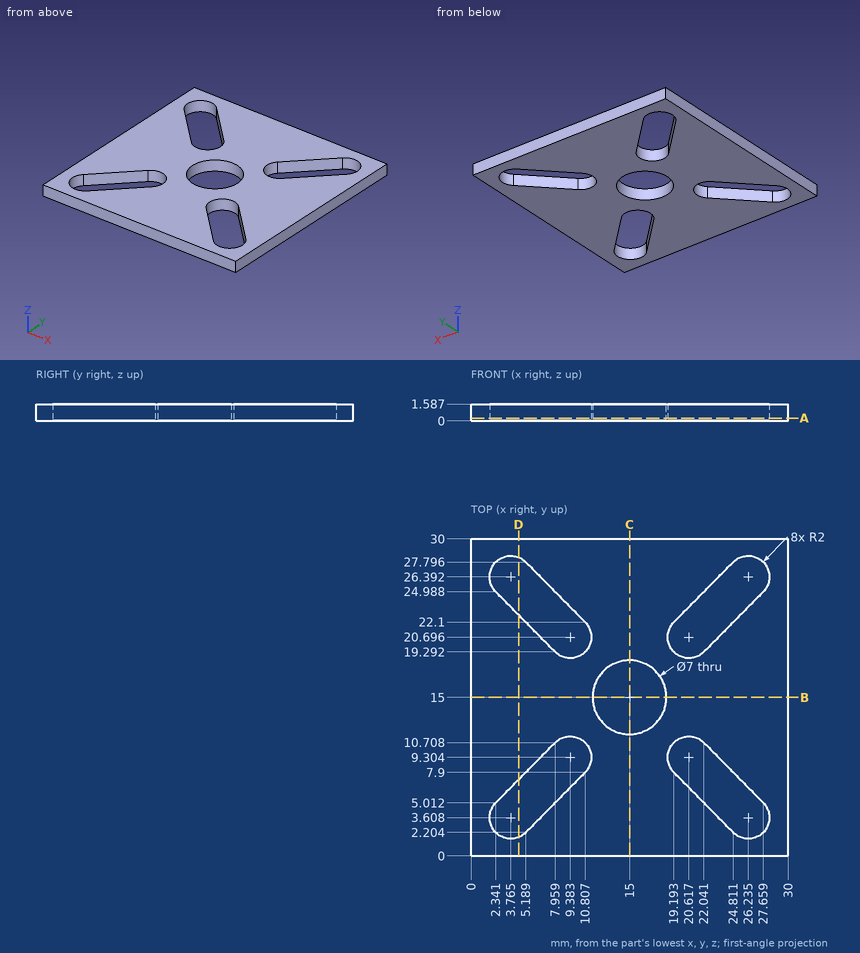
Geometry check sheet. Reference: drawing and pictorial views, mm from the part's lowest x, y, z. Give positions to 0.01 mm unless a question says otherwise; leave off trailing zeros. Write each loop counter-clockwise with the first axis right and the second up, starting at its lowest first coordinate (ties: lowest second). Pieces come first, ordered by that corner, then holes. Notation, with made-up numbers: (45.5, 35) - (58.5, 35) arc R21 ccw to (58.5, 65) - close; hole circle Ø10 at (-32.75, 47). An arc over 180 degrees is marked (long way). Put each result on its own line as item: value.
Q1. Section check B-B on y = 15. Record the cut outline in (x, z).
Result:
outline: (0, 0) - (11.5, 0) - (11.5, 1.59) - (0, 1.59) - close; (18.5, 0) - (30, 0) - (30, 1.59) - (18.5, 1.59) - close
Q2. Scan lines: probe 1 along Y at (x, z) = (15, 0.7); probe 2 along Y at (x, z) = (3.75, 1.45) (1 decimal); probe 3 along X at (y, z) = (9.5, 1.2) (1 decimal). Record each from-to range of solid material in increasing order. Write a range as from..to.
Result:
probe 1: 0..11.5, 18.5..30
probe 2: 0..1.6, 6.4..23.6, 28.4..30
probe 3: 0..6.8, 11.4..18.6, 23.2..30
Q3. Section check D-D on x = 4.5. Record the cut outline in (y, z).
Result:
outline: (0, 0) - (1.75, 0) - (1.75, 1.59) - (0, 1.59) - close; (7.2, 0) - (22.8, 0) - (22.8, 1.59) - (7.2, 1.59) - close; (28.25, 0) - (30, 0) - (30, 1.59) - (28.25, 1.59) - close
Q4. Section check A-A on z = 0.25. Record the cut outline in (x, y) (1 decimal).
Result:
outline: (0, 0) - (30, 0) - (30, 30) - (0, 30) - close; hole (2.3, 5) arc R2 ccw to (5.2, 2.2) - (10.8, 7.9) arc R2 ccw to (8, 10.7) - close; hole (2.3, 25) - (8, 19.3) arc R2 ccw to (10.8, 22.1) - (5.2, 27.8) arc R2 ccw to start; hole circle Ø7 at (15, 15); hole (19.2, 7.9) - (24.8, 2.2) arc R2 ccw to (27.7, 5) - (22, 10.7) arc R2 ccw to start; hole (19.2, 22.1) arc R2 ccw to (22, 19.3) - (27.7, 25) arc R2 ccw to (24.8, 27.8) - close
Q5. Depth check by flat-ended pin: P1, Ø4, axis at x = 11.5, y = 26, coming from the -Z side. Enter the tip coordinate at first touch or a pass-through.
Result:
P1: z = 0
